from build123d import *

# Parameters (mm, degrees)
CROQUIS1_W              = 30
CROQUIS1_H              = 20
SALIENTE_EXTRUIR1_DEPTH = 400
CROQUIS2_R              = 4
CORTAR_EXTRUIR1_DEPTH   = 400


with BuildPart() as part:
    # Croquis1 → Saliente-Extruir1 (new body)
    with BuildSketch(Plane.XY):
        Rectangle(CROQUIS1_W, CROQUIS1_H)
    extrude(amount=SALIENTE_EXTRUIR1_DEPTH)

    # Croquis2 → Cortar-Extruir1 (cut)
    with BuildSketch(Plane(origin=(0, 10, 0), x_dir=(1, 0, 0), z_dir=(0, 1, 0))):
        with Locations((0, -375)):
            Circle(CROQUIS2_R)
        with Locations((0, -25)):
            Circle(CROQUIS2_R)
    extrude(amount=-CORTAR_EXTRUIR1_DEPTH, mode=Mode.SUBTRACT)


solid = part.part
Here's how the part is built. I have some questions about the finished solid (model axes, mm). Coordinates: 2 decimals unless noted, no trailing zeros. Loops run counter-clockwise (first coordinate to the right, second up) from the corner with the lowest first, then second, coordinate; pieces in that order, holes last.
1. For P1, Ø9, axis at x = 0, z = 25, coming from the -Y side, with a flat end and sliding along its axis, tell me the tip position at first contact or that it passes through.
2. Imagine slicing it at B-B, the plane z = 25. Please give me the cut outline in (x, y).
3. Imagine slicing it at A-A, the plane x = 0. Please give me the cut outline in (y, z), and give its area (3 significant figures).
4. If we mould it in two halves opening along Z, with no side actions, what happens to faces 1 (the flat face through (0, -10, 197)), 2 (the flat face through (0, 0, 400)), 3 (the cylindrical face through (-0.521, 0.14, 21.034))? For each: pulls with the +Z half, pulls with the -Z half, needs draft (parallel to the pull), parting line crosses it, or undercut.
5. I need wall thicknesses on L1, parallel to Z at x = 0, y = 5.25; L2, parallel to Z at x = 2.25, y = 3.25; L3, parallel to X at y = 4, z = 25. Which ranges of each line are inside material? Lowest first, please.
Taken from the geometry:
1. P1: stops at y = -10
2. outline: (-15, -10) - (-4, -10) - (-4, 10) - (-15, 10) - close; (4, -10) - (15, -10) - (15, 10) - (4, 10) - close
3. outline: (-10, 0) - (10, 0) - (10, 21) - (-10, 21) - close; (-10, 29) - (10, 29) - (10, 371) - (-10, 371) - close; (-10, 379) - (10, 379) - (10, 400) - (-10, 400) - close
3. area: 7,680 mm2
4. face 1: needs draft
4. face 2: pulls with the +Z half
4. face 3: undercut
5. L1: z = 0 to 21, 29 to 371, 379 to 400
5. L2: z = 0 to 21.69, 28.31 to 371.69, 378.31 to 400
5. L3: x = -15 to -4, 4 to 15
